Geometry check sheet. Reference: the model listing, model coordinates, mm. Face numbers are marked on the shaded views. Coordinates: 2 decimals unless noted, no trailing zeros. Write each loop counter-clockwise with the first axis right and the second up, starting at its lowest first coordinate (ties: lowest second). Pieces come first, ordered by that corner, then holes. Notation, with made-up numbers: M 33.25,9.25 L 76.25,9.25 A5 ccw 76.25,18.25 Z; hole C 57,71.25 d1. An arc over 180 degrees is marked long. Write each question's results on one line, items separated by ' | '.
```python
from build123d import *

# Parameters (mm, degrees)
CROQUIS1_R              = 1.6
SALIENTE_EXTRUIR1_DEPTH = 6
REDONDEO1_R             = 3.727663


with BuildPart() as part:
    # Croquis1 → Saliente-Extruir1 (new body)
    with BuildSketch(Plane.XY):
        with BuildLine():
            Line((-6, 0), (6, 0))
            ThreePointArc((6, 0), (9.5, 3.5), (6, 7))
            Line((6, 7), (4, 15.22))
            Line((4, 15.22), (2.929440389, 19.62))
            Line((2.929440389, 19.62), (-2.929440389, 19.62))
            Line((-2.929440389, 19.62), (-4, 15.22))
            Line((-4, 15.22), (-6, 7))
            ThreePointArc((-6, 7), (-9.5, 3.5), (-6, 0))
        make_face()
        with Locations((6, 3.5)):
            Circle(CROQUIS1_R, mode=Mode.SUBTRACT)
        with Locations((-6, 3.5)):
            Circle(CROQUIS1_R, mode=Mode.SUBTRACT)
        with Locations((0, 17.44)):
            Circle(CROQUIS1_R, mode=Mode.SUBTRACT)
        with Locations((0, 9.9)):
            Circle(CROQUIS1_R, mode=Mode.SUBTRACT)
    extrude(amount=SALIENTE_EXTRUIR1_DEPTH)

    # Redondeo1
    redondeo1_edges = [part.edges().sort_by_distance(p)[0] for p in [
        (-2.929440389, 19.62, 3),
        (2.929440389, 19.62, 3),
    ]]
    fillet(redondeo1_edges, radius=REDONDEO1_R)


solid = part.part
```
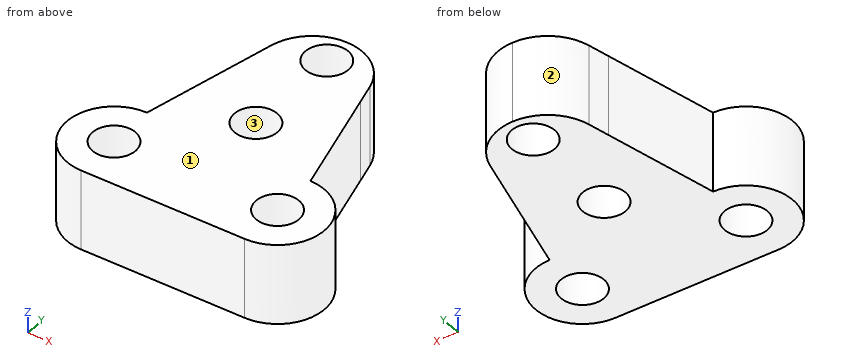
Q1. Mould release check, pull along X, two halves, no side actions. Record for the marked faces 1, 2 and 3: pulls with the +X half, pulls with the -X half, needs draft (parallel to the pull), parting line crosses it, or undercut.
Geometry check:
face 1: needs draft | face 2: pulls with the -X half | face 3: undercut
Q2. Sectioned sample at C-C on x = 1.25. Record the cut outline in (y, z).
Geometry check:
outline: M 0,0 L 8.9,0 L 8.9,6 L 0,6 Z; M 10.9,0 L 16.44,0 L 16.44,6 L 10.9,6 Z; M 18.44,0 L 19.4,0 L 19.4,6 L 18.44,6 Z
Q3. Depth check by flat-ended pin: P1, Ø1.9, axis at x = 0, y = 17.44, coming from the +Z side; P2, Ø2, axis at y = 9.5, z = 1, coming from the +X side. Enter the tip coordinate at first touch or a pass-through.
Geometry check:
P1: passes through | P2: stops at x = 5.64
Q4. Sectioned sample at A-A on z = 1.15. Record the cut outline in (x, y), and give its area (3 significant figures).
Geometry check:
outline: M -6,0 L 6,0 A3.5 ccw 6,7 L 3.62,16.77 A3.73 ccw -3.62,16.77 L -6,7 A3.5 ccw Z; hole C -6,3.5 d3.2; hole C 0,9.9 d3.2; hole C 0,17.44 d3.2; hole C 6,3.5 d3.2 | area: 200 mm2
Q5. Sectioned sample at D-D on y = 17.44. Record the cut outline in (x, z).
Geometry check:
outline: M -3.39,0 L -1.6,0 L -1.6,6 L -3.39,6 Z; M 1.6,0 L 3.39,0 L 3.39,6 L 1.6,6 Z
Q6. Scan lines: probe 1 along X at (y, z) = (2.5, 2.9); probe 2 along X at (y, z) = (4.25, 1.25); probe 3 along X at (y, z) = (16, 2.1). Record each from-to range of solid material in increasing order.
Geometry check:
probe 1: x = -9.35 to -7.25, -4.75 to 4.75, 7.25 to 9.35 | probe 2: x = -9.42 to -7.41, -4.59 to 4.59, 7.41 to 9.42 | probe 3: x = -3.81 to -0.7, 0.7 to 3.81
Q7. Sectioned sample at B-B on y = 3.5. Record the cut outline in (x, z).
Geometry check:
outline: M -9.5,0 L -7.6,0 L -7.6,6 L -9.5,6 Z; M -4.4,0 L 4.4,0 L 4.4,6 L -4.4,6 Z; M 7.6,0 L 9.5,0 L 9.5,6 L 7.6,6 Z
